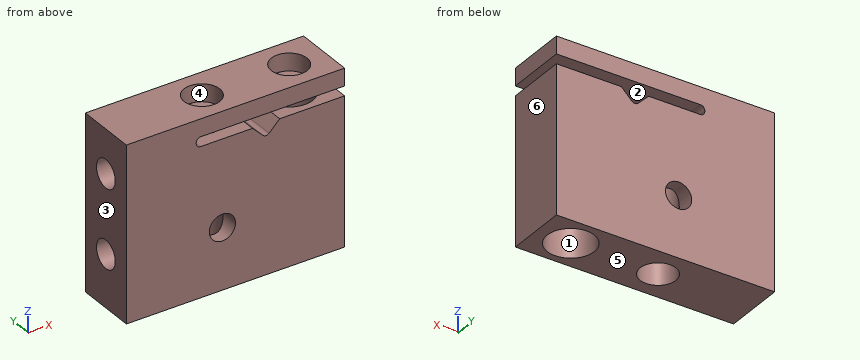
from build123d import *

# Parameters (mm, degrees)
SKETCH1_W                      = 12.5
SKETCH1_H                      = 10
BOSS_EXTRUDE1_DEPTH            = 3.5
CUT_EXTRUDE1_DEPTH             = 3.5
M2_5_CLEARANCE_HOLE1_D         = 2.7
M2_5_CLEARANCE_HOLE1_DEPTH     = 8.45
M2_5_TAPPED_HOLE1_D            = 2.05
M2_5_TAPPED_HOLE1_DEPTH        = 1
F_1_5_1_5_DIAMETER_HOLE1_D     = 1.5
F_1_5_1_5_DIAMETER_HOLE1_DEPTH = 3.5
M2_5_TAPPED_HOLE2_D            = 2.05
M2_TAPPED_HOLE3_D              = 1.6
M2_TAPPED_HOLE3_DEPTH          = 5
M2_TAPPED_HOLE3_TIP            = 0.480688495


with BuildPart() as part:
    # Sketch1 → Boss-Extrude1 (new body)
    with BuildSketch(Plane(origin=(0, 0, 0), x_dir=(1, 0, 0), z_dir=(0, 1, 0))):
        Rectangle(SKETCH1_W, SKETCH1_H)
    extrude(amount=BOSS_EXTRUDE1_DEPTH)

    # Sketch2 → Cut-Extrude1 (cut)
    with BuildSketch(Plane(origin=(0, 3.5, 0), x_dir=(1, 0, 0), z_dir=(0, 1, 0))):
        with BuildLine():
            Line((2.527817459, -3.45), (1.926776695, -2.848959236))
            ThreePointArc((1.926776695, -2.848959236), (1.75, -2.775735931), (1.573223305, -2.848959236))
            Line((1.573223305, -2.848959236), (0.972182541, -3.45))
            Line((0.972182541, -3.45), (-2, -3.45))
            ThreePointArc((-2, -3.45), (-2.176776695, -3.523223305), (-2.25, -3.7))
            Line((-2.25, -3.7), (-2.25, -3.75))
            ThreePointArc((-2.25, -3.75), (-2.176776695, -3.926776695), (-2, -4))
            Line((-2, -4), (6.25, -4))
            Line((6.25, -4), (6.25, -3.45))
            Line((6.25, -3.45), (2.527817459, -3.45))
        make_face()
    extrude(amount=-CUT_EXTRUDE1_DEPTH, mode=Mode.SUBTRACT)

    # M2.5 Clearance Hole1
    with Locations(Plane(origin=(0, 0, -5), x_dir=(-1, 0, 0), z_dir=(0, 0, -1))):
        with Locations((-4.25, 1.75)):
            Hole(M2_5_CLEARANCE_HOLE1_D / 2, depth=M2_5_CLEARANCE_HOLE1_DEPTH)

    # M2.5 Tapped Hole1
    with Locations(Plane.XY.offset(5)):
        with Locations((4.25, 1.75)):
            Hole(M2_5_TAPPED_HOLE1_D / 2, depth=M2_5_TAPPED_HOLE1_DEPTH)

    # Ø1.5 (1.5) Diameter Hole1
    with Locations(Plane(origin=(0, 3.5, 0), x_dir=(1, 0, 0), z_dir=(0, 1, 0))):
        with Locations((-0.75, 1.5)):
            Hole(F_1_5_1_5_DIAMETER_HOLE1_D / 2, depth=F_1_5_1_5_DIAMETER_HOLE1_DEPTH)

    # M2.5 Tapped Hole2 (through all)
    with Locations(Plane(origin=(0, 0, -5), x_dir=(-1, 0, 0), z_dir=(0, 0, -1))):
        with Locations((0.75, 1.75)):
            Hole(M2_5_TAPPED_HOLE2_D / 2)

    # M2 Tapped Hole3
    with Locations(Plane.ZY.offset(6.25)):
        with Locations((-2, 1.75), (2.5, 1.75)):
            Hole(M2_TAPPED_HOLE3_D / 2, depth=M2_TAPPED_HOLE3_DEPTH)
            with Locations((0, 0, -(M2_TAPPED_HOLE3_DEPTH + M2_TAPPED_HOLE3_TIP / 2))):  # 118° drill point
                Cone(0, M2_TAPPED_HOLE3_D / 2, M2_TAPPED_HOLE3_TIP, mode=Mode.SUBTRACT)


solid = part.part
Check sheet for the modelled part. Datum: model origin and axes. Units: mm. Face numbers are marked on the shaded views. A direction names the side the tool comes from. Coordinates: 2 decimals unless noted, no trailing zeros. Write each loop counter-clockwise with the first axis right and the second up, starting at its lowest first coordinate (ties: lowest second). Pieces come first, ordered by that corner, then holes.
Item 1: Cross-section at D-D on z = 4.25. Record the boundary of the cut face in (x, y) (3 decimals).
Numbers:
outline: (-6.25, 0) - (6.25, 0) - (6.25, 3.5) - (-6.25, 3.5) - close; hole circle Ø2.05 at (-0.75, 1.75); hole circle Ø2.05 at (4.25, 1.75)
Item 2: Mould release check, pull along X, two halves, no side actions. Record for the marked faces 4, 5 and 6: released by +X, released by -X, zero draft, split by the parting line, or undercut.
Numbers:
face 4: undercut
face 5: zero draft
face 6: released by +X
Item 3: Cross-section at B-B on z = -2. Record the boundary of the cut face in (x, y) (3 decimals), then the cut area to 3 significant figures.
Numbers:
outline: (-6.25, 0) - (-1.309, 0) - (-1.309, 0.891) arc R1.025 cw to (-1.391, 0.95) - (-6.25, 0.95) - close; (-6.25, 2.55) - (-1.391, 2.55) arc R1.025 cw to (-1.309, 2.609) - (-1.309, 3.5) - (-6.25, 3.5) - close; (-0.191, 0) - (6.25, 0) - (6.25, 3.5) - (-0.191, 3.5) - (-0.191, 2.609) arc R1.025 cw to (-0.191, 0.891) - close; hole circle Ø2.7 at (4.25, 1.75)
area: 25.6 mm2
Item 4: Cross-section at A-A on x = -0.75. Record the boundary of the cut face in (y, z) (3 decimals).
Numbers:
outline: (0, -5) - (0.725, -5) - (0.725, -2.25) - (0, -2.25) - close; (0, -0.75) - (0.725, -0.75) - (0.725, 3.45) - (0, 3.45) - close; (0, 4) - (0.725, 4) - (0.725, 5) - (0, 5) - close; (2.775, -5) - (3.5, -5) - (3.5, -2.25) - (2.775, -2.25) - close; (2.775, -0.75) - (3.5, -0.75) - (3.5, 3.45) - (2.775, 3.45) - close; (2.775, 4) - (3.5, 4) - (3.5, 5) - (2.775, 5) - close
Item 5: Scan lines: probe 1 along Z at (x, y) = (0.5, 0.4); probe 2 along Z at (x, y) = (-0.75, 3.2); probe 3 along Z at (x, y) = (-5.25, 1.5). Record each from-to range of solid material in increasing order.
Numbers:
probe 1: z = -5 to 3.45, 4 to 5
probe 2: z = -5 to -2.25, -0.75 to 3.45, 4 to 5
probe 3: z = -5 to -2.76, -1.24 to 1.74, 3.26 to 5
Item 6: Cross-section at C-C on x = 4.25. Record the boundary of the cut face in (y, z) (3 decimals), then the cut area to 3 significant figures.
Numbers:
outline: (0, -5) - (0.4, -5) - (0.4, 3.45) - (0, 3.45) - close; (0, 4) - (0.725, 4) - (0.725, 5) - (0, 5) - close; (2.775, 4) - (3.5, 4) - (3.5, 5) - (2.775, 5) - close; (3.1, -5) - (3.5, -5) - (3.5, 3.45) - (3.1, 3.45) - close
area: 8.21 mm2
Item 7: Access from +Z, -Z, +X, -X, +Y, -Y to the whole of each face (thin tool, end or side, straight path). Record for the marked faces 1, 2 and 3.
Numbers:
face 1: -Z
face 2: +X, +Y, -Y
face 3: +Z, -Z, -X, +Y, -Y
Item 8: Depth check by flat-ended pin: pin 1 Ø1.5 at (x, y) = (-1.5, 2) entering from +Z. Enter the tip coordinate at first touch or a pass-through.
Numbers:
pin 1: stops at z = 5
